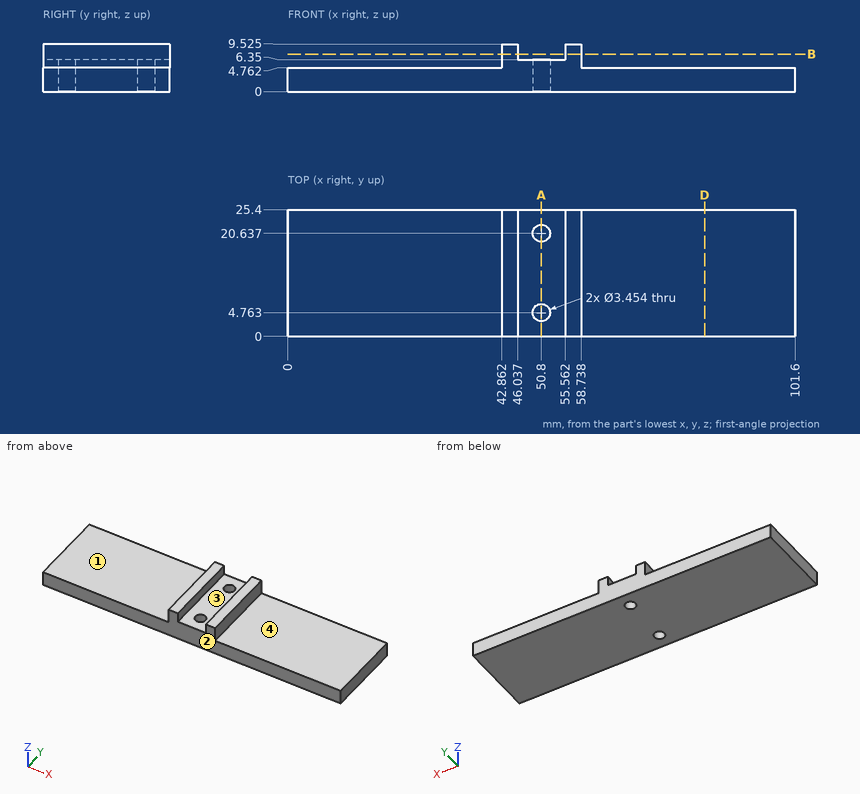
Job drawing, mm, ordinate dimensions from the low corner. One solid piece. A direction names the side the tool comes from. Give positions to 0.01 mm unless a question says otherwise; leave off trailing zeros. Loops run counter-clockwise (first coordinate to the right, second up) from the corner with the lowest first, then second, coordinate; pieces in that order, holes last. Notation, with made-up numbers: M 73,49.25 L 109,49.25 A20 ccw 109,55.25 Z; hole C -38,66 d11. An arc over 180 degrees is marked long. Answer in a Markdown table with one row per item. Add a question column.
Item 1: Probe probe 1 along Y at (x, z) = (50.8, 3.5) (1 decimal); probe 2 along X at (y, z) = (6.5, 6.75); probe 3 along Z at (x, y) = (35, 23.25). List the from-to ranges inside material, lowest first.
Item 2: Band-saw the part on B-B on z = 7.5. Give the cut face in (x, y), then the cut area to 3 significant figures.
Item 3: Band-saw the part on A-A on x = 50.8. Give the number of separate pieces and of enclosed holes in the cut face, then the cut area to 3 significant figures.
Item 4: Band-saw the part on D-D on x = 83.5. Give the cut face in (y, z), then the cut area to 3 significant figures.
Item 5: Tool access for the marked faces 1, 2, 3 and 4: list every direction of +Z, -Z, +X, -X, +Y, -Y with a clear straight run to the whole face (end or side of a thin tool).
Item 6: Drop flat-ended pins along their axis: P1, Ø6, axis at x = 60.5, y = 17.5, coming from the +Z side (1 decimal); P2, Ø3.5, axis at y = 15.5, z = 7, coming from the +X side; P3, Ø2, axis at x = 50.8, y = 4.76, coming from the -Z side; P4, Ø5, axis at x = 50, y = 18, coming from the +Z side. Give the stop position or say it passes through.
Reply:
| question | item | result |
|---|---|---|
| 1 | probe 1 | y = 0 to 3, 6.5 to 18.9, 22.4 to 25.4 |
| 1 | probe 2 | x = 42.86 to 46.04, 55.56 to 58.74 |
| 1 | probe 3 | z = 0 to 4.76 |
| 2 | outline | M 42.86,0 L 46.04,0 L 46.04,25.4 L 42.86,25.4 Z; M 55.56,0 L 58.74,0 L 58.74,25.4 L 55.56,25.4 Z |
| 2 | area | 161 mm^2 |
| 3 | separate pieces | 3 |
| 3 | enclosed holes | 0 |
| 3 | area | 117 mm^2 |
| 4 | outline | M 0,0 L 25.4,0 L 25.4,4.76 L 0,4.76 Z |
| 4 | area | 121 mm^2 |
| 5 | face 1 | +Z, -X, +Y, -Y |
| 5 | face 2 | +Z, -Z, +X, -X, -Y |
| 5 | face 3 | +Z, +Y, -Y |
| 5 | face 4 | +Z, +X, +Y, -Y |
| 6 | P1 | stops at z = 9.5 |
| 6 | P2 | stops at x = 58.74 |
| 6 | P3 | passes through |
| 6 | P4 | stops at z = 6.35 |
